Read the model definition and answer for the solid it produces. Units are mm, in the model's axes. A direction names the side the tool comes from. Give positions to 0.01 mm unless a question says otherwise; leave off trailing zeros. Write each loop counter-clockwise with the first axis right and the second up, starting at its lowest first coordinate (ties: lowest second). Pieces come first, ordered by that corner, then holes. Notation, with made-up numbers: (10, -37.5) -> (23, -37.5) arc R25 ccw to (23, -19.5) -> close; hole circle Ø2 at (50, 74.25). An arc over 180 degrees is marked (long way). Put each result on its own line as item: value. Start each with the question number.
from build123d import *

# Parameters (mm, degrees)
F1_DEPTH = 6.35
F2_R     = 5.08
F3_W     = 12.7
F3_H     = 6.35
F4_DEPTH = 12.7
F3_R     = 1.5875
F5_DEPTH = 127
F6_DEPTH = 31.75


with BuildPart() as f1:
    # F0 (on Right) → F1 (new body, symmetric)
    with BuildSketch(Plane.YZ):
        Polygon((-19.05, 0), (-12.7, 0), (-12.7, 222.25), (12.7, 222.25), (12.7, 0), (19.05, 0), (19.05, 228.6), (12.7, 228.6), (-12.7, 228.6), (-19.05, 228.6), align=None)
    extrude(amount=F1_DEPTH, both=True)

    # F2
    f2_edges = [f1.edges().sort_by_distance(p)[0] for p in [
        (0, -12.7, 222.25),
        (0, 12.7, 222.25),
        (0, -19.05, 228.6),
        (0, 19.05, 228.6),
    ]]
    fillet(f2_edges, radius=F2_R)

    # F3 (on Front) → F4 (join, symmetric)
    with BuildSketch(Plane.XZ):
        with Locations((0, 127)):
            Rectangle(F3_W, F3_H)
    extrude(amount=F4_DEPTH, both=True)

    # F3 (on Front) → F5 (cut, symmetric)
    with BuildSketch(Plane.XZ):
        with Locations((0, 9.525)):
            Circle(F3_R)
    extrude(amount=F5_DEPTH, both=True, mode=Mode.SUBTRACT)

    # F3 (on Front) → F6 (join, symmetric)
    with BuildSketch(Plane.XZ):
        with Locations((0, 9.525)):
            Circle(F3_R)
    extrude(amount=F6_DEPTH, both=True)


solid = f1.part
1) For a pull along Z with two mould halves and no side action, classify faces 1 (the face through (0.089, 11.251, 220.722)), 2 (the face through (0, 19.05, 110)), 3 (the face through (0, 16, 0)), 4 (the face through (-0.089, -17.601, 227.072)) as pulls with the +Z half, pulls with the -Z half, needs draft (parallel to the pull), parting line crosses it, or undercut.
2) Each of these flat-tipped pins is pushed along its axis until it touches: pin 1 Ø5 at (x, z) = (-3, 55.5) entering from -Y; pin 2 Ø3 at (x, z) = (-2.5, 34.5) entering from +Y; pin 3 Ø3 at (y, z) = (21.5, 38.5) entering from -X. Where does it stop, or does it pass through?
3) A cutting plane is placed at A-A on z = 142. Give the vertices of the cut face in (x, y).
4) A cutting plane is placed at B-B on x = 3.5. Give the vertices of the cut face in (y, z) (3 decimals).
5) For faces 5 (the face through (-0.089, 17.522, 227.151)), 6 (the face through (0, -12.7, 173)), determine the directions among +Z, -Z, +X, -X, +Y, -Y from which every point of the face is accessible in a straight line to the end or side of a thin tool.
6) A cutting plane is placed at C-C on y = -24. Give the vertices of the cut face in (x, z) (1 decimal), and give its area (3 significant figures).
7) Straight lines are drawn through the part: line 1 (Z direction, x = -0.25, y = -5) (3 decimals); line 2 (Y direction, x = 2, z = 21). For each, find the intervals that lie inside material, in ascending order. Write a range as [from, to].
Results found:
1. face 1: undercut
1. face 2: needs draft
1. face 3: pulls with the -Z half
1. face 4: pulls with the +Z half
2. pin 1: stops at y = -19.05
2. pin 2: stops at y = 19.05
2. pin 3: passes through
3. outline: (-6.35, -19.05) -> (6.35, -19.05) -> (6.35, -12.7) -> (-6.35, -12.7) -> close; (-6.35, 12.7) -> (6.35, 12.7) -> (6.35, 19.05) -> (-6.35, 19.05) -> close
4. outline: (-19.05, 0) -> (-12.7, 0) -> (-12.7, 123.825) -> (12.7, 123.825) -> (12.7, 0) -> (19.05, 0) -> (19.05, 223.52) arc R5.08 ccw to (13.97, 228.6) -> (-13.97, 228.6) arc R5.08 ccw to (-19.05, 223.52) -> close; hole (-12.7, 130.175) -> (12.7, 130.175) -> (12.7, 217.17) arc R5.08 ccw to (7.62, 222.25) -> (-7.62, 222.25) arc R5.08 ccw to (-12.7, 217.17) -> close
5. face 5: +Z, +X, -X, +Y
5. face 6: +X, -X
6. outline: circle Ø3.2 at (0, 9.5)
6. area: 7.92 mm²
7. line 1: z = [7.957, 11.093], [123.825, 130.175], [222.25, 228.6]
7. line 2: y = [-19.05, -12.7], [12.7, 19.05]
